Job drawing, mm, ordinate dimensions from the low corner. One solid piece. A direction names the side the tool comes from. Give positions to 0.01 mm unless a question says otherwise; leave off trailing zeros. Write each loop counter-clockwise with the first axis right and the second up, starting at its lowest first coordinate (ties: lowest second). Pieces come first, ordered by that corner, then holes. Notation, with made-up numbers: (63, -17) -> (86, -17) arc R12 cw to (86, -1) -> close; hole circle Ø8 at (20.25, 64.25). An arc over 180 degrees is marked (long way). Put each result on its own line as item: value. Start each with the question number.
Item 1: Two-plate mould, pull along Z, no slides. Class the marked faces 3, 4, 5 and 6: pulls with the +Z half, pulls with the -Z half, needs draft (parallel to the pull), parting line crosses it, or undercut.
Item 2: Tool access for the marked faces 1 and 2: list every direction of +Z, -Z, +X, -X, +Y, -Y with a clear straight run to the whole face (end or side of a thin tool).
Item 3: Flat gauge pins, fed straight in: pin 1 Ø1 at (x, y) = (2.5, 13) entering from -Z; pin 2 Ø2 at (y, z) = (14.5, 7.5) entering from +X. Where does each tip first touch, or does it go through?
Item 4: Slice it at A-A, the plane z = 7.5. List the corners of the cut face in (x, y), plus the area to 3 significant figures.
Item 5: Slice it at D-D, the plane x = 2.3. List the corners of the cut face in (y, z).
Item 6: Slice it at C-C, the plane x = 0.3. List the corners of the cut face in (y, z), plus the area to 3 significant figures.
Item 7: Slice it at B-B, the plane y = 4.5. List the corners of the cut face in (x, z).
Item 8: Drill centre lines: line 1 along Y through (x, z) = (0.6, 7.5); line 2 along Z through (x, y) = (1.45, 4.5); line 3 along Y through (x, z) = (3.3, 7.5). Where is each one in solid material? Low to high.
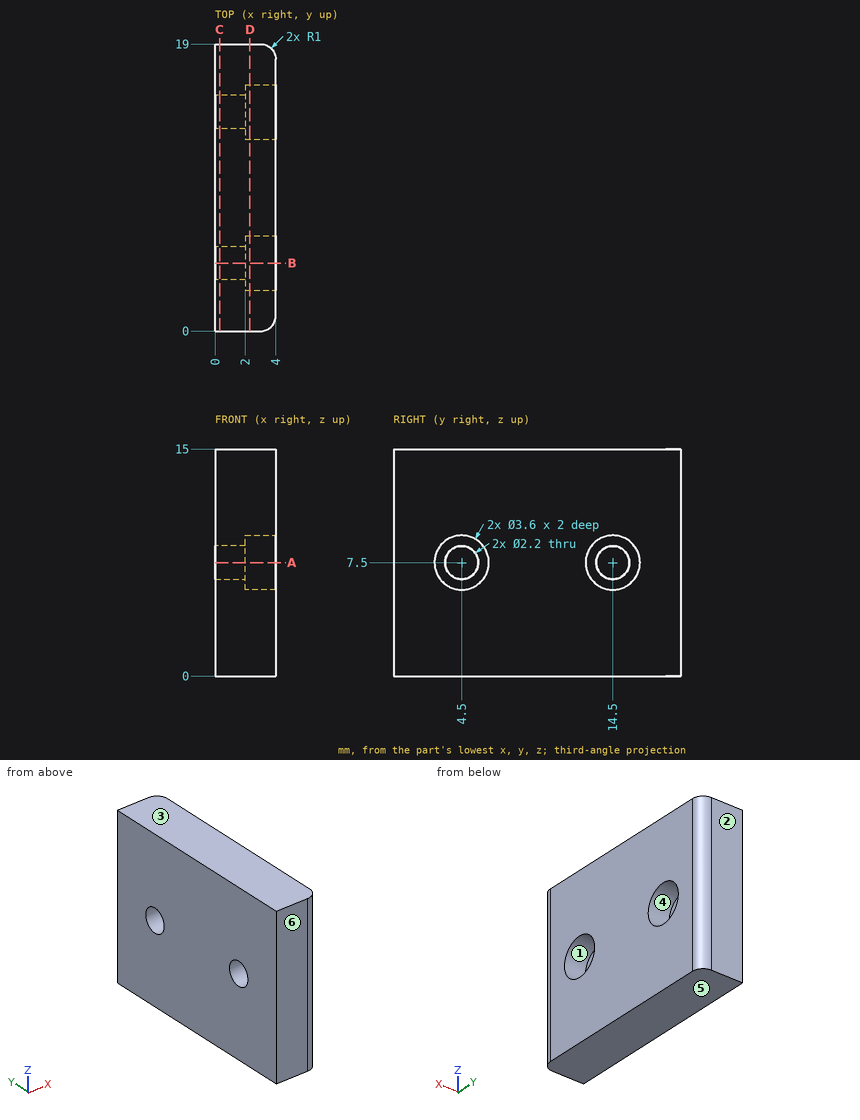
Values follow:
1. face 3: pulls with the +Z half
1. face 4: undercut
1. face 5: pulls with the -Z half
1. face 6: needs draft
2. face 1: +X
2. face 2: +Z, -Z, +X, -X, +Y
3. pin 1: z = 0
3. pin 2: through
4. outline: (0, 0) -> (3, 0) arc R1 ccw to (4, 1) -> (4, 2.7) -> (2, 2.7) -> (2, 3.4) -> (0, 3.4) -> close; (0, 5.6) -> (2, 5.6) -> (2, 6.3) -> (4, 6.3) -> (4, 12.7) -> (2, 12.7) -> (2, 13.4) -> (0, 13.4) -> close; (0, 15.6) -> (2, 15.6) -> (2, 16.3) -> (4, 16.3) -> (4, 18) arc R1 ccw to (3, 19) -> (0, 19) -> close
4. area: 52.4 mm2
5. outline: (0, 0) -> (19, 0) -> (19, 15) -> (0, 15) -> close; hole circle Ø3.6 at (4.5, 7.5); hole circle Ø3.6 at (14.5, 7.5)
6. outline: (0, 0) -> (19, 0) -> (19, 15) -> (0, 15) -> close; hole circle Ø2.2 at (4.5, 7.5); hole circle Ø2.2 at (14.5, 7.5)
6. area: 277 mm2
7. outline: (0, 0) -> (4, 0) -> (4, 5.7) -> (2, 5.7) -> (2, 6.4) -> (0, 6.4) -> close; (0, 8.6) -> (2, 8.6) -> (2, 9.3) -> (4, 9.3) -> (4, 15) -> (0, 15) -> close
8. line 1: 0 to 3.4, 5.6 to 13.4, 15.6 to 19
8. line 2: 0 to 6.4, 8.6 to 15
8. line 3: 0.05 to 2.7, 6.3 to 12.7, 16.3 to 18.95
